For this review, take the finished solid that the model builds, in its own axes (mm). Face numbers are marked on the shaded views. A direction names the side the tool comes from. Coordinates: 2 decimals unless noted, no trailing zeros. Write each loop counter-clockwise with the first axis right and the second up, starting at its lowest first coordinate (ties: lowest second). Pieces come first, ordered by that corner, then holes. Notation, with made-up numbers: (64, 22) -> (92, 22) arc R25 ccw to (92, 60) -> close; hole circle Ø11 at (-9, 79.5). An arc over 180 degrees is marked (long way). One line per item, written item: value. Start each with the question number.
1) Machinability: for the marked faces 5, 6 and 7, which of the approach directions +Z, -Z, +X, -X, +Y, -Y give a long, thin tool a straight path to every point of the face, cutting with its end or side? Answer none if there is none.
2) Add section C-C (y = 26). State the section outline as (x, z) points.
3) Mouldability with a two-part tool opening along Y and no side actions: class the marked faces 1, 2, 3 and 4 as released by +Y, released by -Y, zero draft, split by the parting line, or undercut.
4) For pin 1 Ø12 at (y, z) = (-0.5, -20.5) entering from -X; pin 2 Ø3 at (y, z) = (19.5, 0) entering from +X; pin 3 Ø3 at (x, z) = (18.5, -21) entering from -Y, all flat-tipped, find the tip position at first contact; note any pin that passes through.
5) For probe 1 along X at (y, z) = (5, 17.5); probe 2 along X at (y, z) = (25, -4); probe 3 along Z at (x, y) = (25, 1), list the stretches that pass through material, from the lowest coordinate up. Write a range as from..to.
6) Add section A-A (x = 14.75). State the section outline as (y, z) points, and give its area (3 significant figures).
from build123d import *

# Parameters (mm, degrees)
F3_DEPTH = 25
F4_SIZE  = 3
F5_R     = 30.5581123827
F5_R_2   = 17
F6_DEPTH = 1


with BuildPart() as f1:
    # F0 (on Front) → F1 (revolve)
    with BuildSketch(Plane.XZ):
        with BuildLine():
            Line((0, 17), (0, 0))
            Line((0, 0), (11, 0))
            ThreePointArc((11, 0), (15.5551164444, 8.914228848), (25.4479047191, 10.4456667115))
            Line((25.4479047191, 10.4456667115), (27.5, 14))
            Line((27.5, 14), (27.5, 17))
            Line((27.5, 17), (23, 17))
            Line((23, 17), (23, 16))
            Line((23, 16), (21, 16))
            Line((21, 16), (21, 17))
            Line((21, 17), (18.5, 17))
            Line((18.5, 17), (18.5, 40))
            Line((18.5, 40), (14, 40))
            Line((14, 40), (14, 17))
            Line((14, 17), (0, 17))
        make_face()
    revolve(axis=Axis((11, 0, 0), (1, 0, 0)))

    # F2 (on face) → F3 (cut)
    with BuildSketch(Plane(origin=(14, 0, 0), x_dir=(0, -1, 0), z_dir=(-1, 0, 0))):
        with BuildLine():
            ThreePointArc((16.8416654415, -36.281652459), (20, -34.6410161514), (23, -32.7261363439))
            Line((23, -32.7261363439), (23, -13.2790561914))
            Line((23, -13.2790561914), (0, -26.5581123827))
            Line((0, -26.5581123827), (16.8416654415, -36.281652459))
        make_face()
        with BuildLine():
            Line((23, -13.2790561914), (23, -32.7261363439))
            ThreePointArc((23, -32.7261363439), (34.6410161514, -20), (39.8416654415, -3.5555161151))
            Line((39.8416654415, -3.5555161151), (23, -13.2790561914))
        make_face()
        with BuildLine():
            Line((23, 13.2790561914), (23, -13.2790561914))
            Line((23, -13.2790561914), (39.8416654415, -3.5555161151))
            ThreePointArc((39.8416654415, -3.5555161151), (39.9603967552, -1.7795199266), (40, 0))
            ThreePointArc((40, 0), (39.9603967552, 1.7795199266), (39.8416654415, 3.5555161151))
            Line((39.8416654415, 3.5555161151), (23, 13.2790561914))
        make_face()
        with BuildLine():
            Line((23, 32.7261363439), (23, 13.2790561914))
            Line((23, 13.2790561914), (39.8416654415, 3.5555161151))
            ThreePointArc((39.8416654415, 3.5555161151), (34.6410161514, 20), (23, 32.7261363439))
        make_face()
        with BuildLine():
            Line((0, 26.5581123827), (23, 13.2790561914))
            Line((23, 13.2790561914), (23, 32.7261363439))
            ThreePointArc((23, 32.7261363439), (20, 34.6410161514), (16.8416654415, 36.281652459))
            Line((16.8416654415, 36.281652459), (0, 26.5581123827))
        make_face()
        with BuildLine():
            Line((-16.8416654415, 36.281652459), (0, 26.5581123827))
            Line((0, 26.5581123827), (16.8416654415, 36.281652459))
            ThreePointArc((16.8416654415, 36.281652459), (0, 40), (-16.8416654415, 36.281652459))
        make_face()
        with BuildLine():
            Line((-23, 13.2790561914), (0, 26.5581123827))
            Line((0, 26.5581123827), (-16.8416654415, 36.281652459))
            ThreePointArc((-16.8416654415, 36.281652459), (-20, 34.6410161514), (-23, 32.7261363439))
            Line((-23, 32.7261363439), (-23, 13.2790561914))
        make_face()
        with BuildLine():
            Line((-39.8416654415, -3.5555161151), (-23, -13.2790561914))
            Line((-23, -13.2790561914), (-23, 13.2790561914))
            Line((-23, 13.2790561914), (-39.8416654415, 3.5555161151))
            ThreePointArc((-39.8416654415, 3.5555161151), (-40, 0), (-39.8416654415, -3.5555161151))
        make_face()
        with BuildLine():
            Line((-23, -32.7261363439), (-23, -13.2790561914))
            Line((-23, -13.2790561914), (-39.8416654415, -3.5555161151))
            ThreePointArc((-39.8416654415, -3.5555161151), (-34.6410161514, -20), (-23, -32.7261363439))
        make_face()
        with BuildLine():
            Line((-16.8416654415, -36.281652459), (0, -26.5581123827))
            Line((0, -26.5581123827), (-23, -13.2790561914))
            Line((-23, -13.2790561914), (-23, -32.7261363439))
            ThreePointArc((-23, -32.7261363439), (-20, -34.6410161514), (-16.8416654415, -36.281652459))
        make_face()
        with BuildLine():
            ThreePointArc((-16.8416654415, -36.281652459), (0, -40), (16.8416654415, -36.281652459))
            Line((16.8416654415, -36.281652459), (0, -26.5581123827))
            Line((0, -26.5581123827), (-16.8416654415, -36.281652459))
        make_face()
        with BuildLine():
            Line((-39.8416654415, 3.5555161151), (-23, 13.2790561914))
            Line((-23, 13.2790561914), (-23, 32.7261363439))
            ThreePointArc((-23, 32.7261363439), (-34.6410161514, 20), (-39.8416654415, 3.5555161151))
        make_face()
    extrude(amount=-F3_DEPTH, mode=Mode.SUBTRACT)

    # F4
    f4_edges = [f1.edges().sort_by_distance(p)[0] for p in [
        (0, 0, -17),
    ]]
    chamfer(f4_edges, length=F4_SIZE)

    # F5 (on face) → F6 (join)
    with BuildSketch(Plane.YZ.offset(18.5)):
        Circle(F5_R)
        Polygon((23, 13.2790561914), (23, -13.2790561914), (0, -26.5581123827), (-23, -13.2790561914), (-23, 13.2790561914), (0, 26.5581123827), align=None, mode=Mode.SUBTRACT)
        Polygon((0, -26.5581123827), (23, -13.2790561914), (23, 13.2790561914), (0, 26.5581123827), (-23, 13.2790561914), (-23, -13.2790561914), align=None)
        Circle(F5_R_2, mode=Mode.SUBTRACT)
    extrude(amount=F6_DEPTH)


solid = f1.part
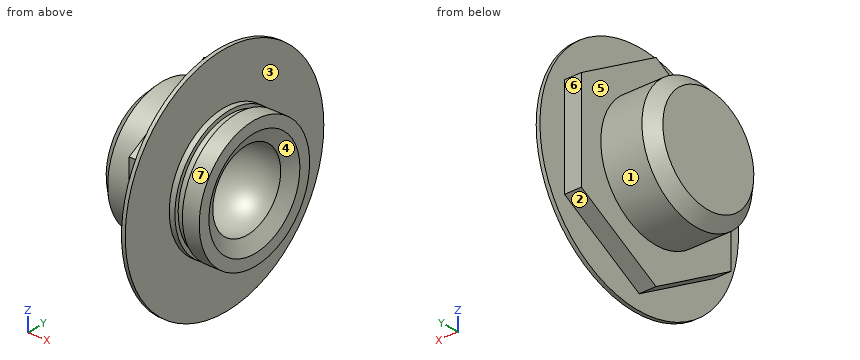
Numbers:
1. face 5: -X
1. face 6: +Z, -Z, -X, +Y
1. face 7: +X
2. outline: (18.5, -16.06) -> (19.5, -16.06) -> (19.5, 16.06) -> (18.5, 16.06) -> close
3. face 1: split by the parting line
3. face 2: released by +Y
3. face 3: zero draft
3. face 4: undercut
4. pin 1: x = 0.51
4. pin 2: x = 19.5
4. pin 3: y = -23.53
5. probe 1: 14..19.5
5. probe 2: 18.5..19.5
5. probe 3: -16.97..-10.54, 10.54..16.97
6. outline: (-23, -13.28) -> (0, -26.56) -> (23, -13.28) -> (23, 13.28) -> (0, 26.56) -> (-23, 13.28) -> close; hole circle Ø16.55 at (0, 0)
6. area: 1,620 mm²
